```python
from build123d import *

# Parameters (mm, degrees)
F0_W      = 135
F0_H      = 85
F1_DEPTH  = 2
F2_W      = 131.53
F2_H      = 82
F2_W_2    = 128.53
F2_H_2    = 79
F3_DEPTH  = 3.38
F4_SIZE2  = 0.3464101615
F4_SIZE   = 0.2
F5_R      = 0.3
F6_W      = 4
F6_H      = 73
F7_DEPTH  = 25
F8_DEPTH  = 1
F9_DEPTH  = 1
F10_W     = 128.53
F10_H     = 5
F11_DEPTH = 5.38


with BuildPart() as f1:
    # F0 (on Top) → F1 (new body)
    with BuildSketch(Plane.XY):
        Rectangle(F0_W, F0_H)
    extrude(amount=F1_DEPTH)

    # F2 (on face) → F3 (join)
    with BuildSketch(Plane.XY.offset(2)):
        Rectangle(F2_W, F2_H)
        Rectangle(F2_W_2, F2_H_2, mode=Mode.SUBTRACT)
    extrude(amount=F3_DEPTH)

    # F4
    f4_edges = [f1.edges().sort_by_distance(p)[0] for p in [
        (-65.765, 0, 5.38),
        (0, 41, 5.38),
        (0, -41, 5.38),
        (65.765, 0, 5.38),
    ]]
    f4_side = f1.faces().sort_by_distance((0, 40.845003, 5.38))[0]
    chamfer(f4_edges, length=F4_SIZE, length2=F4_SIZE2, reference=f4_side)

    # F5
    f5_edges = [f1.edges().sort_by_distance(p)[0] for p in [
        (65.765, 0, 5.03359),
        (0, 41, 5.03359),
        (0, -41, 5.03359),
        (-65.765, 0, 5.03359),
    ]]
    fillet(f5_edges, radius=F5_R)

    # F6 (on face) → F7 (cut)
    with BuildSketch(Plane.XY.offset(2)):
        with Locations((-59.265, 0)):
            Rectangle(F6_W, F6_H)
        with Locations((-51.265, 0)):
            Rectangle(F6_W, F6_H)
        with Locations((-43.265, 0)):
            Rectangle(F6_W, F6_H)
        with Locations((-35.265, 0)):
            Rectangle(F6_W, F6_H)
        with Locations((-27.265, 0)):
            Rectangle(F6_W, F6_H)
        with Locations((-19.265, 0)):
            Rectangle(F6_W, F6_H)
        with Locations((-11.265, 0)):
            Rectangle(F6_W, F6_H)
        with Locations((-3.265, 0)):
            Rectangle(F6_W, F6_H)
        with Locations((35.265, 0)):
            Rectangle(F6_W, F6_H)
        with Locations((43.265, 0)):
            Rectangle(F6_W, F6_H)
        with Locations((51.265, 0)):
            Rectangle(F6_W, F6_H)
        with Locations((3.265, 0)):
            Rectangle(F6_W, F6_H)
        with Locations((59.265, 0)):
            Rectangle(F6_W, F6_H)
        with Locations((11.265, 0)):
            Rectangle(F6_W, F6_H)
        with Locations((19.265, 0)):
            Rectangle(F6_W, F6_H)
        with Locations((27.265, 0)):
            Rectangle(F6_W, F6_H)
    extrude(amount=-F7_DEPTH, mode=Mode.SUBTRACT)

    # F8 (cut): a face of the model
    f8_faces = [f1.faces().sort_by_distance(p)[0] for p in [
        (0, 0, 0),
    ]]
    extrude(f8_faces, amount=-F8_DEPTH, mode=Mode.SUBTRACT)

    # F9 (add): a face of the model
    f9_faces = [f1.faces().sort_by_distance(p)[0] for p in [
        (0, 0, 1),
    ]]
    extrude(f9_faces, amount=F9_DEPTH)

    # F10 (on face) → F11 (join, through all)
    with BuildSketch(Plane.XY.offset(5.38)):
        Rectangle(F10_W, F10_H)
    extrude(amount=-F11_DEPTH)


solid = f1.part
```
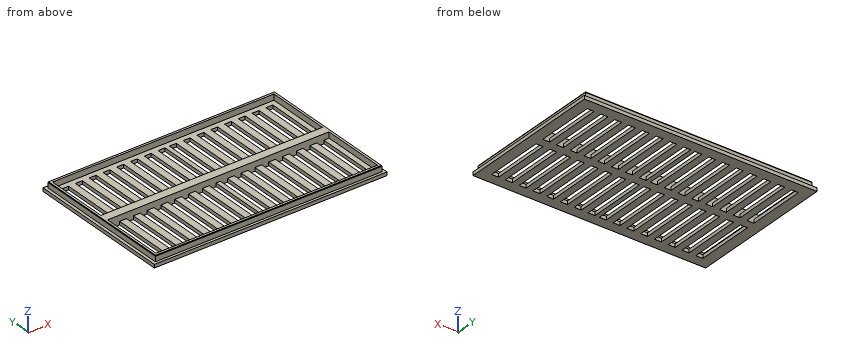
Source: CAD feature listing. Evaluate the final solid. Frame: model axes, mm. Give positions to 0.01 mm unless a question says otherwise; leave off trailing zeros. Loops run counter-clockwise (first coordinate to the right, second up) from the corner with the lowest first, then second, coordinate; pieces in that order, holes last. Notation, with made-up numbers: (-7.75, 4.5) - (39.25, 4.5) arc R24 ccw to (39.25, 27.5) - close; hole circle Ø3 at (44.5, 10). An arc over 180 degrees is marked (long way). Use CSV: the item, a comma, the result in double quotes. Start each with the question number.
1. Section A-A (z = 2.85). Output: boundary loops of the cut face in (x, y) (3 decimals).
2. Pin query (flat end, axial travel): pin 1 (0.9 mm diameter, centred on y = -2.5, z = 4, fed in from +X) (3 decimals); pin 2 (3 mm diameter, centred on y = 17, z = 4.5, fed in from -X) (3 decimals); pin 3 (3 mm diameter, centred on x = 42.5, y = -19, fed in from -Z); pin 4 (3 mm diameter, centred on x = 16.5, z = 4, fed in from +Y). Return the tip coordinate at first contact, or that it passes through.
3. Section D-D (y = -23.5). Count the separate pieces of the cut face and the enclosed holes in it, then the cut area to 3 significant figures.
4. Section C-C (y = 0.5). Output: boundary loops of the cut face in (x, z) (3 decimals), then the cut area to 4 significant figures.
5. Section B-B (x = -39). Output: boundary loops of the cut face in (y, z), then the cut area to 3 significant figures.
6. Ray query, L1, parallel to Y at x = -41.5, z = 3.65; L2, parallel to Y at x = 42.5, z = 0.75; L3, parallel to X at y = 30.5, z = 2.65 (3 decimals). Return the intervals inside material, ascending.
Response:
1,outline,"(-65.765, -41) - (65.765, -41) - (65.765, 41) - (-65.765, 41) - close; hole (-64.265, -39.5) - (64.265, -39.5) - (64.265, -2.5) - (-64.265, -2.5) - close; hole (-64.265, 2.5) - (64.265, 2.5) - (64.265, 39.5) - (-64.265, 39.5) - close"
2,pin 1,"x = 65.765"
2,pin 2,"x = -65.765"
2,pin 3,"z = 0"
2,pin 4,"y = 41"
3,separate pieces,"17"
3,enclosed holes,"0"
3,area,"152 mm²"
4,outline,"(-67.5, 0) - (67.5, 0) - (67.5, 2) - (65.765, 2) - (65.765, 4.953) arc R0.3 ccw to (65.725, 5.103) - (65.565, 5.38) - (-65.565, 5.38) - (-65.725, 5.103) arc R0.3 ccw to (-65.765, 4.953) - (-65.765, 2) - (-67.5, 2) - close"
4,area,"714.5 mm²"
5,outline,"(-42.5, 0) - (42.5, 0) - (42.5, 2) - (41, 2) - (41, 4.95) arc R0.3 ccw to (40.96, 5.1) - (40.8, 5.38) - (39.5, 5.38) - (39.5, 2) - (2.5, 2) - (2.5, 5.38) - (-2.5, 5.38) - (-2.5, 2) - (-39.5, 2) - (-39.5, 5.38) - (-40.8, 5.38) - (-40.96, 5.1) arc R0.3 ccw to (-41, 4.95) - (-41, 2) - (-42.5, 2) - close"
5,area,"197 mm²"
6,L1,"-41 to -39.5, -2.5 to 2.5, 39.5 to 41"
6,L2,"-42.5 to -36.5, -2.5 to 2.5, 36.5 to 42.5"
6,L3,"-65.765 to -64.265, 64.265 to 65.765"
